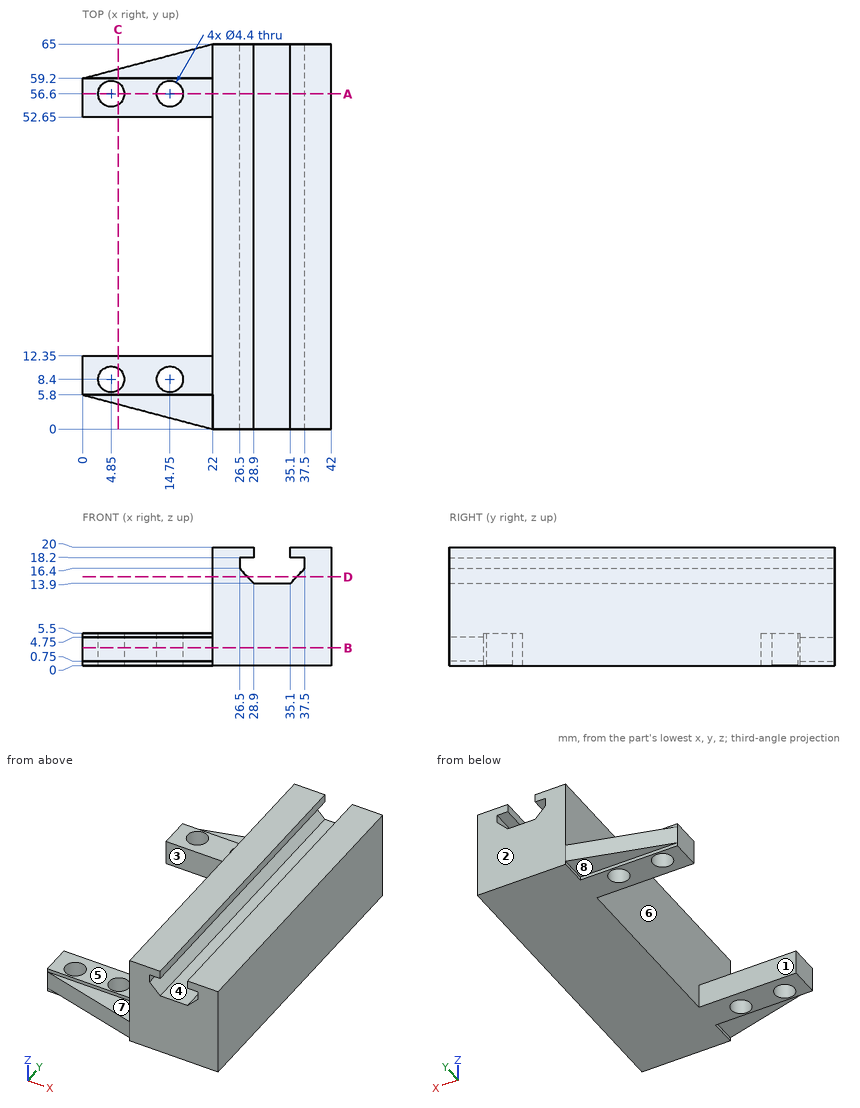
Geometry: see drawing. Coordinates: mm, zero at the bounding-box minimum. A direction names the side the tool comes from. Give positions to 0.01 mm unless a question says otherwise; leave off trailing zeros. Write each loop counter-clockwise with the first axis right and the second up, starting at its lowest first coordinate (ties: lowest second). Pieces come first, ordered by that corner, then holes. Notation, with made-up numbers: M -7.5,34 L -2.5,34 A24 ccw -2.5,57 Z; hole C 84.5,14.5 d10. An arc over 180 degrees is marked long. Answer in a Markdown table with one row per item. Add a question column.
(1) Section B-B on z = 3. Return loops of the section in (x, y), and give its area (3 significant figures).
(2) Section C-C on x = 6. Return loops of the section in (y, z).
(3) First-contact query: pin 1 (10 mm diameter, centred on x = 16.5, y = 7.5, fed in from +Z); pin 2 (1.2 mm diameter, centred on x = 27.5, y = 29.5, fed in from -Z); pin 3 (8 mm diameter, centred on x = 16, z = 5, fed in from -Y); pin 4 (1.7 mm diameter, centred on x = 14.5, y = 62.5, fed in from -Z). Flat tips, straight axial feed; report the tip coordinate or a pass-through.
(4) Section D-D on z = 15. Return loops of the section in (x, y).
(5) Mould query, pull axis Y, two halves, no side actions, for the marked faces 1, 2, 3 and 4. Classes: +Y half, -Y half, draft (parallel to the pull), parting line (faces both ways), or undercut.
(6) Section A-A on y = 56.6. Return loops of the section in (x, z).
(7) Reachability of the marked faces 5, 6, 7 and 8 from +Z, -Z, +X, -X, +Y, -Y: full face, straight path, thin tool, end or side. Return the list, or none.
(8) Ray query, line 1 (Y direction, x = 4.85, z = 3.2); line 2 (Y direction, x = 14.75, z = 3.6); line 3 (Z direction, x = 6.5, y = 10). Return the intervals inside material, ascending.
Result set:
| question | item | result |
|---|---|---|
| 1 | outline | M 0,5.8 L 22,0 L 42,0 L 42,65 L 22,65 L 0,59.2 L 0,52.65 L 22,52.65 L 22,12.35 L 0,12.35 Z; hole C 4.85,8.4 d4.4; hole C 4.85,56.6 d4.4; hole C 14.75,8.4 d4.4; hole C 14.75,56.6 d4.4 |
| 1 | area | 1,650 mm^2 |
| 2 | outline | M 4.22,0.75 L 5.8,0.75 L 5.8,0 L 6.52,0 L 6.52,5.5 L 5.8,5.5 L 5.8,4.75 L 4.22,4.75 Z; M 10.28,0 L 12.35,0 L 12.35,5.5 L 10.28,5.5 Z; M 52.65,0 L 54.72,0 L 54.72,5.5 L 52.65,5.5 Z; M 58.48,0 L 59.2,0 L 59.2,0.75 L 60.78,0.75 L 60.78,4.75 L 59.2,4.75 L 59.2,5.5 L 58.48,5.5 Z |
| 3 | pin 1 | stops at z = 5.5 |
| 3 | pin 2 | stops at z = 0 |
| 3 | pin 3 | stops at y = 0.53 |
| 3 | pin 4 | stops at z = 0.75 |
| 4 | outline | M 22,0 L 27.84,0 L 27.84,65 L 22,65 Z; M 36.16,0 L 42,0 L 42,65 L 36.16,65 Z |
| 5 | face 1 | undercut |
| 5 | face 2 | +Y half |
| 5 | face 3 | undercut |
| 5 | face 4 | draft |
| 6 | outline | M 0,0 L 2.65,0 L 2.65,5.5 L 0,5.5 Z; M 7.05,0 L 12.55,0 L 12.55,5.5 L 7.05,5.5 Z; M 16.95,0 L 42,0 L 42,20 L 35.1,20 L 35.1,18.2 L 37.5,18.2 L 37.5,16.4 L 35.1,13.9 L 28.9,13.9 L 26.5,16.4 L 26.5,18.2 L 28.9,18.2 L 28.9,20 L 22,20 L 22,5.5 L 16.95,5.5 Z |
| 7 | face 5 | +Z, -X, +Y, -Y |
| 7 | face 6 | +Z, -X |
| 7 | face 7 | +Z, -X, -Y |
| 7 | face 8 | -Z, -X, +Y |
| 8 | line 1 | y = 4.52 to 6.2, 10.6 to 12.35, 52.65 to 54.4, 58.8 to 60.48 |
| 8 | line 2 | y = 1.91 to 6.2, 10.6 to 12.35, 52.65 to 54.4, 58.8 to 63.09 |
| 8 | line 3 | z = 0 to 5.5 |
